Autodesk Inventor part; units mm, degrees
ref_plane "YZ Plane" through (0, 0, 0) normal (1, 0, 0) x (0, 1, 0)
ref_plane "XZ Plane" through (0, 0, 0) normal (0, 1, 0) x (-1, 0, 0)
ref_plane "XY Plane" through (0, 0, 0) normal (0, 0, 1) x (1, 0, 0)
sketch "Sketch3" plane through (0, 0, 0) normal (0, 0, 1) x (1, 0, 0)
  line L0 (-10, 20) -> (-20, 15)
  line L1 (-10, 20) -> (-27.4665, 29.933)
  line L2 (-27.4665, 29.933) -> (-27.4665, 73.9793)
  line L3 (-27.4665, 73.9793) -> (-17.4665, 73.9793)
  line L4 (-17.4665, 73.9793) -> (-10, 34.7248)
  line L5 (10, 20) -> (20, 15)
  line L6 (10, 20) -> (27.4665, 29.933)
  line L7 (27.4665, 29.933) -> (27.4665, 73.9793)
  line L8 (27.4665, 73.9793) -> (17.4665, 73.9793)
  line L9 (17.4665, 73.9793) -> (10, 34.7248)
  circle A0 centre (-22.4665, 63.181) radius 2.5
  circle A1 centre (-22.4665, 42.2172) radius 2.5
  circle A2 centre (22.4665, 63.181) radius 2.5
  circle A3 centre (22.4665, 42.2172) radius 2.5
  arc A4 (-10, 34.7248) -> (10, 34.7248) centre (0, 40.7878) ccw
  line L10 (-20, 15) -> (-20, 10)
  line L11 (-20, 10) -> (-15, 10)
  line L12 (-15, 10) -> (-15, 0)
  line L13 (-15, 0) -> (15, 0)
  line L14 (15, 0) -> (15, 10)
  line L15 (15, 10) -> (20, 10)
  line L16 (20, 10) -> (20, 15)
  point P0 (0, 0)
  dimension "d2" = 10
  dimension "d3" = 5
  dimension "d4" = 5
  dimension "d9" = 5
  dimension "d10" = 5
  dimension "d11" = 30
  dimension "d12" = 90
  dimension "d13" = 5
extrude "Extrusion1" add sketch "Sketch3" along normal blind 5.5
fillet "Fillet1" radius 2 4 edges at (27.4665, 29.933, 2.75) (-27.4665, 29.933, 2.75) (-10, 20, 2.75) (10, 20, 2.75)
properties part number "sables"
Geometry: final body of the model. Coordinates: model frame, mm. A direction names the side the tool comes from. Give positions to 0.01 mm unless a question says otherwise; leave off trailing zeros. Write each loop counter-clockwise with the first axis right and the second up, starting at its lowest first coordinate (ties: lowest second). Pieces come first, ordered by that corner, then holes. Notation, with made-up numbers: (-24, 21.5) -> (-8, 21.5) arc R24 cw to (-8, 35.5) -> close; hole circle Ø9 at (74.25, 41.5). An arc over 180 degrees is marked (long way). Answer in a Markdown table with one row per item.
(1) Section query C-C on y = 52. Return loops of the section in (x, z).
Answers below:
| item | result |
|---|---|
| outline | (-27.47, 0) -> (-13.29, 0) -> (-13.29, 5.5) -> (-27.47, 5.5) -> close; (13.29, 0) -> (27.47, 0) -> (27.47, 5.5) -> (13.29, 5.5) -> close |
(2) Draft query along X for faces 4 (the flat face through (0, 0, 3)), 5 (the cylindrical face through (-23.008, 44.658, 2.712)), 6 (the flat face through (-19.76, 25.55, 2.71)), 7 (the flat face through (20, 12, 3)). Return one class per face: +X half, -X half, draft (parallel to the pull), parting line (faces both ways), or undercut.
Answers below:
| item | result |
|---|---|
| face 4 | draft |
| face 5 | undercut |
| face 6 | -X half |
| face 7 | +X half |
(3) Section query A-A on y = 43.5. Return loops of the section in (x, z), then the cut area to 3 significant figures.
Answers below:
| item | result |
|---|---|
| outline | (-27.47, 0) -> (-24.61, 0) -> (-24.61, 5.5) -> (-27.47, 5.5) -> close; (-20.32, 0) -> (-11.67, 0) -> (-11.67, 5.5) -> (-20.32, 5.5) -> close; (11.67, 0) -> (20.32, 0) -> (20.32, 5.5) -> (11.67, 5.5) -> close; (24.61, 0) -> (27.47, 0) -> (27.47, 5.5) -> (24.61, 5.5) -> close |
| area | 127 mm^2 |
(4) Ray query, line 1 along Y through (x, z) = (-22, 1.15); line 2 along X through (y, z) = (62.5, 3.85); line 3 along X through (y, z) = (44.5, 1.1). Return the intervals inside material, ascending. Write a range as [from, to].
Answers below:
| item | result |
|---|---|
| line 1 | [26.82, 39.76], [44.67, 60.72], [65.64, 73.98] |
| line 2 | [-27.47, -24.87], [-20.06, -15.28], [15.28, 20.06], [24.87, 27.47] |
| line 3 | [-27.47, -23.49], [-21.45, -11.86], [11.86, 21.45], [23.49, 27.47] |
(5) Section query D-D on x = -22. Return loops of the section in (y, z).
Answers below:
| item | result |
|---|---|
| outline | (26.82, 0) -> (39.76, 0) -> (39.76, 5.5) -> (26.82, 5.5) -> close; (44.67, 0) -> (60.72, 0) -> (60.72, 5.5) -> (44.67, 5.5) -> close; (65.64, 0) -> (73.98, 0) -> (73.98, 5.5) -> (65.64, 5.5) -> close |
(6) Pin query (flat end, axial travel): pin 1 (2.5 mm diameter, centred on x = 18, z = 3, fed in from -Y); pin 2 (1.6 mm diameter, centred on y = 6.5, z = 1.5, fed in from +X); pin 3 (8 mm diameter, centred on x = 14.5, y = 26, fed in from -Z); pin 4 (1.5 mm diameter, centred on y = 11.5, z = 3, fed in from +X). Return the tip coordinate at first contact, or that it passes through.
Answers below:
| item | result |
|---|---|
| pin 1 | y = 10 |
| pin 2 | x = 15 |
| pin 3 | z = 0 |
| pin 4 | x = 20 |
(7) Section query B-B on x = -16.5. Return loops of the section in (y, z).
Answers below:
| item | result |
|---|---|
| outline | (10, 0) -> (16.75, 0) -> (16.75, 5.5) -> (10, 5.5) -> close; (23.7, 0) -> (68.9, 0) -> (68.9, 5.5) -> (23.7, 5.5) -> close |
(8) Set-up query: faces 1 (the flat face through (16.6, 16.7, 2.7)), 2 (the flat face through (-13.786, 54.627, 2.712)), 3 (the flat face through (-16.6, 16.7, 2.7)). Return all of +Z, -Z, +X, -X, +Y, -Y with unobstructed straight access to the full face (end or side cutting, diameter ignored); none if empty.
Answers below:
| item | result |
|---|---|
| face 1 | +Z, -Z, +X |
| face 2 | +Z, -Z, +Y |
| face 3 | +Z, -Z, -X |
